Can you work these out from the drawing? Everything is in mm from the part's minimum corner. Coordinates: 2 decimals unless noted, no trailing zeros. Write each loop counter-clockwise with the first axis right and the second up, starting at its lowest first coordinate (ties: lowest second). Pieces come first, ordered by that corner, then holes. Notation, with made-up numbers: (-1.75, -6) -> (42.25, -6) arc R10 ccw to (42.25, 0) -> close; hole circle Ø3 at (-30.75, 60). An arc over 180 degrees is marked (long way). Use CSV: the item, a comma, the result in double quotes. Start each with the question number.
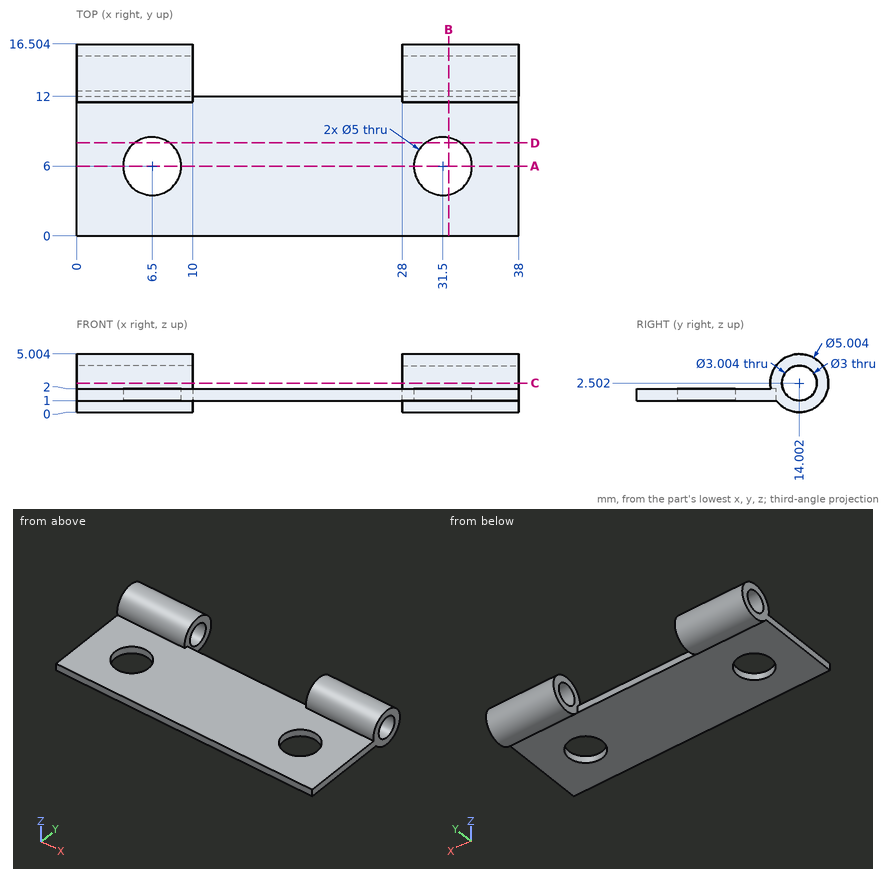
Item 1: I want a section at B-B on x = 32. Count the separate pieces of the cut face and the enclosed holes in it, then the cut area to 3 significant figures.
Item 2: I want a section at D-D on y = 8. Please give me the cut outline in (x, z).
Item 3: I want a section at C-C on z = 2.5. Please give me the cut outline in (x, y).
Item 4: I want a section at A-A on y = 6. Please give me the cut outline in (x, z), then the cut area to 3 significant figures.
Item 5: If I drill on line 1 along X through (y, z) = (14.5, 0.95); line 2 along Y through (x, z) = (31.5, 1.7); line 3 along Z through (x, y) = (34, 0.5), over which ranges is the centre line in solid material (lowest first)?
Item 6: I'm going to push flat-ended pins straight in: pin 1 (1.5 mm diameter, centred on x = 26.5, y = 9, fed in from +Z); pin 2 (1.1 mm diameter, centred on x = 12.5, z = 1.5, fed in from +Y); pin 3 (4 mm diameter, centred on x = 31, y = 7, fed in from -Z). Where does each tip first touch, or does it pass through?
Geometry says:
1,separate pieces,"2"
1,enclosed holes,"1"
1,area,"19.4 mm2"
2,outline,"(0, 1) -> (5, 1) -> (5, 2) -> (0, 2) -> close; (8, 1) -> (30, 1) -> (30, 2) -> (8, 2) -> close; (33, 1) -> (38, 1) -> (38, 2) -> (33, 2) -> close"
3,outline,"(0, 11.5) -> (10, 11.5) -> (10, 12.5) -> (0, 12.5) -> close; (0, 15.5) -> (10, 15.5) -> (10, 16.5) -> (0, 16.5) -> close; (28, 11.5) -> (38, 11.5) -> (38, 12.5) -> (28, 12.5) -> close; (28, 15.5) -> (38, 15.5) -> (38, 16.5) -> (28, 16.5) -> close"
4,outline,"(0, 1) -> (4, 1) -> (4, 2) -> (0, 2) -> close; (9, 1) -> (29, 1) -> (29, 2) -> (9, 2) -> close; (34, 1) -> (38, 1) -> (38, 2) -> (34, 2) -> close"
4,area,"28.0 mm2"
5,line 1,"0 to 10, 28 to 38"
5,line 2,"0 to 3.5, 8.5 to 12.73, 15.27 to 16.37"
5,line 3,"1 to 2"
6,pin 1,"z = 2"
6,pin 2,"y = 12"
6,pin 3,"z = 1"
